```python
from build123d import *

# Parameters (mm, degrees)
BOSS_EXTRUDE1_DEPTH = 5.08
CUT_EXTRUDE1_REACH  = 13.817
SKETCH2_R           = 5.08


with BuildPart() as part:
    # Sketch1 → Boss-Extrude1 (new body)
    with BuildSketch(Plane.XY):
        Polygon((8.065583261, 0), (4.03279163, 6.985), (-4.03279163, 6.985), (-8.065583261, 0), (-4.03279163, -6.985), (4.03279163, -6.985), align=None)
    extrude(amount=BOSS_EXTRUDE1_DEPTH)

    # Sketch2 → Cut-Extrude1 (cut, up to next)
    with BuildSketch(Plane.XY.offset(5.08), mode=Mode.PRIVATE) as cut_extrude1_sk1:
        Circle(SKETCH2_R)
    cut_extrude1_tool1 = extrude(cut_extrude1_sk1.sketch, amount=-CUT_EXTRUDE1_REACH, mode=Mode.PRIVATE) & part.part
    add(cut_extrude1_tool1.solids().sort_by_distance((0, 0, 5.08))[0], mode=Mode.SUBTRACT)


solid = part.part
```
The listing builds one solid part. Answer for the finished solid, in the listing's coordinates (mm). Round coordinates to 2 decimals unless told otherwise and drop trailing zeros. Loops run counter-clockwise (first coordinate to the right, second up) from the corner with the lowest first, then second, coordinate; pieces in that order, holes last.
Q1. Section A-A, the plane x = 0 is taken. Determine the outline of the cut face in (y, z) (3 decimals), then the cut area to 3 significant figures.
Q2. Section D-D, the plane y = -6 is taken. Determine the outline of the cut face in (x, z), then the cut area to 3 significant figures.
Q3. Section B-B, the plane y = -1.25 is taken. Determine the outline of the cut face in (x, z).
Q4. Section C-C, the plane z = 4.2 is taken. Determine the outline of the cut face in (x, y) (3 decimals), then the cut area to 3 significant figures.
Q5. For a pull along Y with two mould halves and no side action, classify faces 1 (the face through (-0.661, 5.037, 2.576)), 2 (the face through (5.3, 0.1, 5.08)), 3 (the face through (0, 6.985, 3)) as released by +Y, released by -Y, zero draft, split by the parting line, or undercut.
Q6. Find the intervals of material crossed by line 1 (Y direction, x = 0, z = 2.65) (3 decimals); line 2 (Y direction, x = 2, z = 2.5) (3 decimals); line 3 (X direction, y = -2.75, z = 2.9), in increasing order.
Q7. Given pin 1 Ø1.5 at (y, z) = (-0.5, 3) entering from -X; pin 2 Ø3 at (x, y) = (3.5, 0.5) entering from +Z; pin 3 Ø3 at (y, z) = (2, 2.5) entering from -X, each flat-ended and moving along its own axis, determine where each tip first touches the part or whether it passes through.
Completed:
1. outline: (-6.985, 0) - (-5.08, 0) - (-5.08, 5.08) - (-6.985, 5.08) - close; (5.08, 0) - (6.985, 0) - (6.985, 5.08) - (5.08, 5.08) - close
1. area: 19.4 mm2
2. outline: (-4.6, 0) - (4.6, 0) - (4.6, 5.08) - (-4.6, 5.08) - close
2. area: 46.8 mm2
3. outline: (-7.34, 0) - (-4.92, 0) - (-4.92, 5.08) - (-7.34, 5.08) - close; (4.92, 0) - (7.34, 0) - (7.34, 5.08) - (4.92, 5.08) - close
4. outline: (-8.066, 0) - (-4.033, -6.985) - (4.033, -6.985) - (8.066, 0) - (4.033, 6.985) - (-4.033, 6.985) - close; hole circle Ø10.16 at (0, 0)
4. area: 87.9 mm2
5. face 1: undercut
5. face 2: zero draft
5. face 3: released by +Y
6. line 1: y = -6.985 to -5.08, 5.08 to 6.985
6. line 2: y = -6.985 to -4.67, 4.67 to 6.985
6. line 3: x = -6.48 to -4.27, 4.27 to 6.48
7. pin 1: stops at x = -8.07
7. pin 2: passes through
7. pin 3: stops at x = -7.78
